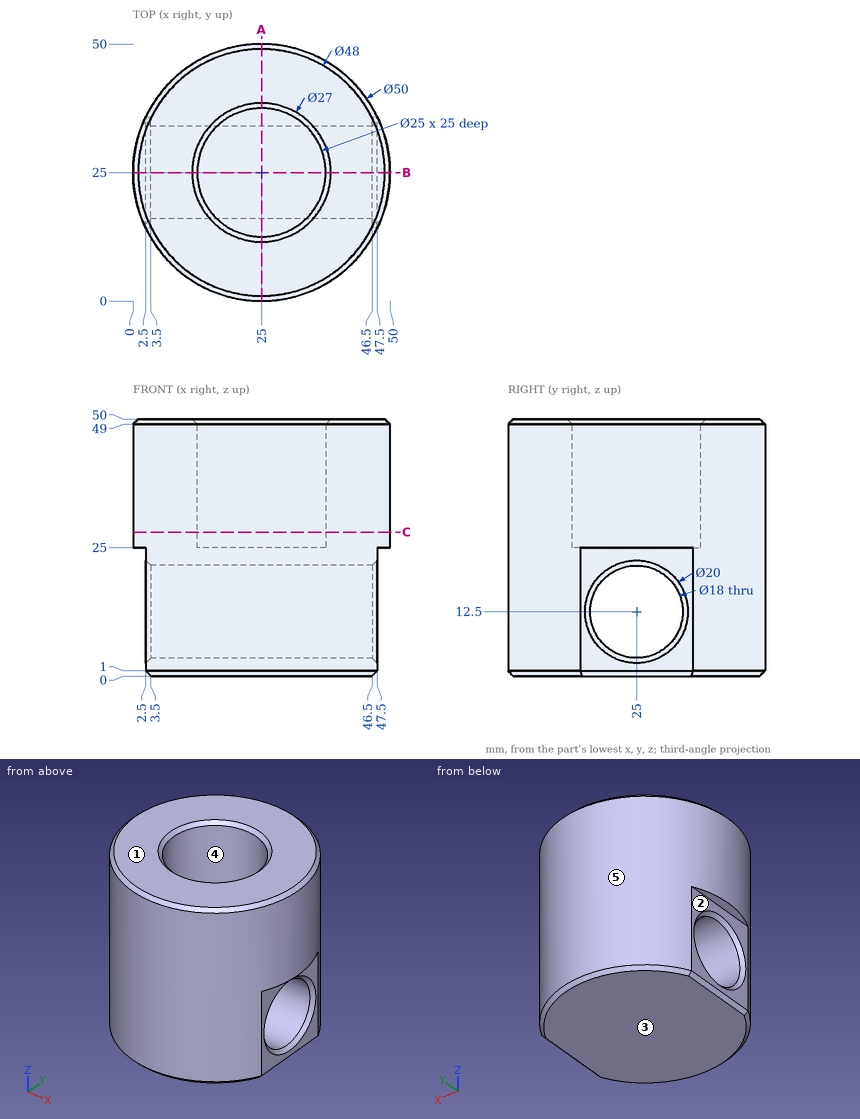
Study the drawing (mm; zero at the part's minimum x, y, z) and answer. A direction names the side the tool comes from. Coordinates: 2 decimals unless noted, no trailing zeros. Loops run counter-clockwise (first coordinate to the right, second up) from the corner with the lowest first, then second, coordinate; pieces in that order, holes last. Notation, with made-up numbers: M -27,58.5 L 22,58.5 A22 ccw 22,83.5 Z; hole C 38.25,-34 d8. An arc over 180 degrees is marked long. Answer in a Markdown table with one row per item.
1) Find section A-A (x = 25). Determine the outline of the cut face in (y, z).
Answers below:
| item | result |
|---|---|
| outline | M 0,1 L 1,0 L 49,0 L 50,1 L 50,49 L 49,50 L 38.5,50 L 37.5,49 L 37.5,25 L 12.5,25 L 12.5,49 L 11.5,50 L 1,50 L 0,49 Z; hole C 25,12.5 d18 |
2) Determine the mould class of the marked faces 3, 4 and 5 for opening direction Y: released by +Y, released by -Y, zero draft, split by the parting line, or undercut.
Answers below:
| item | result |
|---|---|
| face 3 | zero draft |
| face 4 | undercut |
| face 5 | split by the parting line |
3) Find section B-B (y = 25). Determine the outline of the cut face in (x, z).
Answers below:
| item | result |
|---|---|
| outline | M 0,25 L 2.5,25 L 2.5,22.5 L 3.5,21.5 L 46.5,21.5 L 47.5,22.5 L 47.5,25 L 50,25 L 50,49 L 49,50 L 38.5,50 L 37.5,49 L 37.5,25 L 12.5,25 L 12.5,49 L 11.5,50 L 1,50 L 0,49 Z; M 2.5,1 L 3.5,0 L 46.5,0 L 47.5,1 L 47.5,2.5 L 46.5,3.5 L 3.5,3.5 L 2.5,2.5 Z |
4) Find section C-C (z = 28). Determine the outline of the cut face in (x, y), then the cut area to 3 significant figures.
Answers below:
| item | result |
|---|---|
| outline | C 25,25 d50; hole C 25,25 d25 |
| area | 1,470 mm^2 |
5) Given pin 1 (2 mm diameter, centred on y = 12.5, z = 20, fed in from -X); pin 2 (8 mm diameter, centred on x = 21, z = 39, fed in from +Y); pin 3 (2 mm diameter, centred on x = 31.5, z = 20, fed in from +Y), each flat-ended and moving along its own axis, determine where each tip first touches the part or whether it passes through.
Answers below:
| item | result |
|---|---|
| pin 1 | x = 2.8 |
| pin 2 | y = 50 |
| pin 3 | y = 49.39 |
6) Which of the six approach directions +Z, -Z, +X, -X, +Y, -Y give full straight-line access (tool end or side, diameter ignored) to the marked faces 1 and 2?
Answers below:
| item | result |
|---|---|
| face 1 | +Z, +X, -X, +Y, -Y |
| face 2 | -Z, -X, +Y, -Y |
7) Find the intervals of material crossed by probe 1 along Z at (x, y) = (36, 25); probe 2 along Y at (x, z) = (25, 37.5); probe 3 along Y at (x, z) = (18, 12), in increasing order.
Answers below:
| item | result |
|---|---|
| probe 1 | 0 to 3.5, 21.5 to 25 |
| probe 2 | 0 to 12.5, 37.5 to 50 |
| probe 3 | 1 to 16.01, 33.99 to 49 |
